```python
from build123d import *

# Parameters (mm, degrees)
SKETCH7_R           = 5.7
BOSS_EXTRUDE2_DEPTH = 1
SKETCH8_R           = 5.5
BOSS_EXTRUDE3_DEPTH = 4.5
FILLET4_R           = 0.2
SKETCH9_W           = 5
SKETCH9_H           = 5
BOSS_EXTRUDE4_DEPTH = 0.1
SHELL3_T            = -0.6


with BuildPart() as part:
    # Sketch7 → Boss-Extrude2 (new body)
    with BuildSketch(Plane(origin=(0, 0, 0), x_dir=(1, 0, 0), z_dir=(0, 1, 0))):
        with Locations(Location((0, 0, 0), (0, 0, 270))):
            Circle(SKETCH7_R)
    extrude(amount=BOSS_EXTRUDE2_DEPTH)

    # Sketch8 → Boss-Extrude3 (add)
    with BuildSketch(Plane(origin=(0, 1, 0), x_dir=(1, 0, 0), z_dir=(0, 1, 0))):
        with Locations(Location((0, 0, 0), (0, 0, 270))):
            Circle(SKETCH8_R)
    extrude(amount=BOSS_EXTRUDE3_DEPTH)

    # Fillet4
    fillet4_edges = [part.edges().sort_by_distance(p)[0] for p in [
        (0, 5.5, -5.5),
    ]]
    fillet(fillet4_edges, radius=FILLET4_R)

    # Sketch9 → Boss-Extrude4 (add)
    with BuildSketch(Plane.XZ):
        Rectangle(SKETCH9_W, SKETCH9_H)
    extrude(amount=BOSS_EXTRUDE4_DEPTH)

    # Shell3
    shell3_openings = [part.faces().sort_by_distance(p)[0] for p in [
        (0, -0.1, 0),
    ]]
    offset(amount=SHELL3_T, openings=shell3_openings, kind=Kind.INTERSECTION)


solid = part.part
```
Part model, mm, in its own coordinate system. A direction names the side the tool comes from. Give positions to 0.01 mm unless a question says otherwise; leave off trailing zeros. Write each loop counter-clockwise with the first axis right and the second up, starting at its lowest first coordinate (ties: lowest second). Pieces come first, ordered by that corner, then holes. Notation, with made-up numbers: (-19.5, 55.25) -> (14.5, 55.25) arc R27 cw to (14.5, 87.25) -> close; hole circle Ø10 at (11, -4.5). An arc over 180 degrees is marked (long way). Put each result on its own line as item: value. Start each with the question number.
Item 1: Cut at A-A (y = 0.3). List the corners of the cut face in (x, z), then the cut area to 3 significant figures.
Item 2: Pull direction X, two halves, no side cores. Call faces 4 (the face through (1.472, 2.72, 4.674)), 5 (the face through (-2.3, -0.1, 0)), 6 (the face through (-3.5, 0.5, -4.5)): pulls with the +X half, pulls with the -X half, needs draft (parallel to the pull), parting line crosses it, or undercut.
Item 3: Cut at C-C (x = 0). List the corners of the cut face in (y, z).
Item 4: Which spindle directions (+Z, -Z, +X, -X, +Y, -Y) get a long thin tool onto all of the face, cutting with end or side? Do faces 1 (the face through (-5.37, 3.12, -1.19)), 2 (the face through (0, 5.5, 0)), 3 (the face through (0, 4.9, 0)). Say none if no direction does.
Item 5: Cut at D-D (y = 4.6). List the corners of the cut face in (x, z), then the cut area to 3 significant figures.
Item 6: Wall check: L1, parallel to Y at x = -3, z = -1.5; L2, parallel to Y at x = -2, z = 1.25; L3, parallel to X at y = 2.95, z = 0. Give the ranges that are in metal, low to high. Write a range as [from, to].
Item 7: Pin check, flat tips, straight feed: pin 1 Ø1.5 at (y, z) = (4, 0.5) entering from +X; pin 2 Ø2 at (x, y) = (-1, 3.5) entering from +Z; pin 3 Ø1.5 at (x, y) = (-2.5, 0.5) entering from -Z. Stop position of each tip, or through.
Item 8: Cut at B-B (z = 0). List the corners of the cut face in (x, y).
Answer list:
1. outline: circle Ø11.4 at (0, 0); hole (-1.9, -1.9) -> (1.9, -1.9) -> (1.9, 1.9) -> (-1.9, 1.9) -> close
1. area: 87.6 mm2
2. face 4: undercut
2. face 5: needs draft
2. face 6: parting line crosses it
3. outline: (-0.1, -2.5) -> (0, -2.5) -> (0, -5.7) -> (1, -5.7) -> (1, -5.5) -> (5.3, -5.5) arc R0.2 ccw to (5.5, -5.3) -> (5.5, 5.3) arc R0.2 ccw to (5.3, 5.5) -> (1, 5.5) -> (1, 5.7) -> (0, 5.7) -> (0, 2.5) -> (-0.1, 2.5) -> (-0.1, 1.9) -> (0.6, 1.9) -> (0.6, 4.9) -> (4.9, 4.9) -> (4.9, -4.9) -> (0.6, -4.9) -> (0.6, -1.9) -> (-0.1, -1.9) -> close
4. face 1: +Y
4. face 2: +Z, -Z, +X, -X, +Y
4. face 3: none
5. outline: circle Ø11 at (0, 0); hole circle Ø9.8 at (0, 0)
5. area: 19.6 mm2
6. L1: y = [0, 0.6], [4.9, 5.5]
6. L2: y = [-0.1, 0.6], [4.9, 5.5]
6. L3: x = [-5.5, -4.9], [4.9, 5.5]
7. pin 1: stops at x = 5.5
7. pin 2: stops at z = 5.5
7. pin 3: stops at z = -5.42
8. outline: (-5.7, 0) -> (-2.5, 0) -> (-2.5, -0.1) -> (-1.9, -0.1) -> (-1.9, 0.6) -> (-4.9, 0.6) -> (-4.9, 4.9) -> (4.9, 4.9) -> (4.9, 0.6) -> (1.9, 0.6) -> (1.9, -0.1) -> (2.5, -0.1) -> (2.5, 0) -> (5.7, 0) -> (5.7, 1) -> (5.5, 1) -> (5.5, 5.3) arc R0.2 ccw to (5.3, 5.5) -> (-5.3, 5.5) arc R0.2 ccw to (-5.5, 5.3) -> (-5.5, 1) -> (-5.7, 1) -> close
